```python
from build123d import *
from OCP.BRepFilletAPI import BRepFilletAPI_MakeChamfer

# Parameters (mm, degrees)
SKETCH1_R           = 3.96875
BOSS_EXTRUDE1_DEPTH = 12.7
SKETCH2_R           = 3.96875
CUT_EXTRUDE1_DEPTH  = 4.7625
SKETCH3_R           = 2.5796875
CUT_EXTRUDE2_DEPTH  = 34.474321177
CHAMFER1_SIZE       = 8.89
CHAMFER1_SIZE2      = 3.235695383


with BuildPart() as part:
    # Sketch1 → Boss-Extrude1 (new body)
    with BuildSketch(Plane(origin=(0, 0, 0), x_dir=(1, 0, 0), z_dir=(0, 1, 0))):
        Polygon((0, 0), (27.305, 0), (27.305, 19.3802), (0, 19.3802), (0, 14.6177), (14.605, 14.6177), (14.605, 4.7625), (0, 4.7625), align=None)
        with Locations(Location((20.955, 9.6901, 0), (0, 0, 270))):
            Circle(SKETCH1_R, mode=Mode.SUBTRACT)
    extrude(amount=BOSS_EXTRUDE1_DEPTH)

    # Sketch2 → Cut-Extrude1 (cut)
    with BuildSketch(Plane.XY):
        with Locations((6.985, 6.35)):
            Circle(SKETCH2_R)
    extrude(amount=-CUT_EXTRUDE1_DEPTH, mode=Mode.SUBTRACT)

    # Sketch3 → Cut-Extrude2 (cut, through all)
    with BuildSketch(Plane.XY.offset(-14.6177)):
        with Locations((6.985, 6.35)):
            Circle(SKETCH3_R)
    extrude(amount=-CUT_EXTRUDE2_DEPTH, mode=Mode.SUBTRACT)

    # Chamfer1: one chamfer whose edges measure the first distance from different faces: ONE call of the kernel's chamfer builder (chamfer() names one face for all edges)
    chamfer1_edges_1 = [part.edges().sort_by_distance(p)[0] for p in [
        (27.305, 6.35, -19.3802),
    ]]
    chamfer1_side_1 = [part.faces().sort_by_distance(p)[0] for p in [
        (14.080266617, 6.35, -19.3802),
    ]]
    chamfer1_edges_2 = [part.edges().sort_by_distance(p)[0] for p in [
        (27.305, 6.35, 0),
    ]]
    chamfer1_side_2 = [part.faces().sort_by_distance(p)[0] for p in [
        (14.762286847, 6.35, 0),
    ]]
    chamfer1 = BRepFilletAPI_MakeChamfer(part.part.solid().wrapped)
    for e in chamfer1_edges_1:
        chamfer1.Add(CHAMFER1_SIZE, CHAMFER1_SIZE2, e.wrapped, chamfer1_side_1[0].wrapped)  # the first distance lies on this face
    for e in chamfer1_edges_2:
        chamfer1.Add(CHAMFER1_SIZE, CHAMFER1_SIZE2, e.wrapped, chamfer1_side_2[0].wrapped)  # the first distance lies on this face
    add(Compound.cast(chamfer1.Shape()), mode=Mode.REPLACE)


solid = part.part
```
The listing builds one solid part. Answer for the finished solid, in the listing's coordinates (mm). A direction names the side the tool comes from. Give positions to 0.01 mm unless a question says otherwise; leave off trailing zeros. Order: outer loops, then holes, each group sorted by start corner. A loop starts at its lowest first (then second) coordinate and runs counter-clockwise, first axis right, second up. Notation, with made-up numbers: M -29,44 L -21,44 A22 ccw -21,65 Z; hole C -24.75,23.5 d5. An arc over 180 degrees is marked long. Put each result on its own line as item: value. Start each with the question number.
Item 1: The part is cut by section D-D, the plane x = 4. Determine the outline of the cut face in (y, z).
Item 2: For a pull along Y with two mould halves and no side action, classify faces 3 (the face through (10.77, 7.54, -2.35)), 4 (the face through (16, 0, -10)), 5 (the face through (9.3, 4.8, -19.38)) as +Y half, -Y half, draft (parallel to the pull), parting line (faces both ways), or undercut.
Item 3: The part is cut by section A-A, the plane y = 8.25. Determine the outline of the cut face in (x, z) (1 decimal).
Item 4: Which of the six approach directions +Z, -Z, +X, -X, +Y, -Y give full straight-line access (tool end or side, diameter ignored) to faces 1 (the face through (22.92, 6.26, -1.64)), 2 (the face through (7.2, 9.1, -14.618))?
Item 5: The part is cut by section B-B, the plane z = -8.75. Determine the outline of the cut face in (x, y) (3 decimals).
Item 6: Flat-ended cylindrical pins translate along their axes: P1, Ø3, axis at y = 7.5, z = -4, coming from the -X side; P2, Ø7, axis at x = 20.96, z = -9.69, coming from the +Y side; P3, Ø3, axis at y = 4, z = -12, coming from the -X side (3 decimals). Find the tip coordinate at first contact, or state that the pin passes through.
Item 7: Find the intervals of material crossed by line 1 along Z through (x, y) = (3.5, 2.5); line 2 along X through (y, z) = (3.75, -7.25) (3 decimals); line 3 along Z through (x, y) = (18, 8.25), in increasing order.
Answer key:
1. outline: M 0,-19.38 L 12.7,-19.38 L 12.7,-14.62 L 0,-14.62 Z; M 0,-4.76 L 3.73,-4.76 L 3.73,0 L 0,0 Z; M 8.97,-4.76 L 12.7,-4.76 L 12.7,0 L 8.97,0 Z
2. face 3: undercut
2. face 4: -Y half
2. face 5: draft
3. outline: M 0,-19.4 L 5.2,-19.4 L 5.2,-14.6 L 0,-14.6 Z; M 0,-4.8 L 3.5,-4.8 L 3.5,0 L 0,0 Z; M 8.7,-19.4 L 18.4,-19.4 L 27.3,-16.1 L 27.3,-3.2 L 18.4,0 L 10.5,0 L 10.5,-4.8 L 14.6,-4.8 L 14.6,-14.6 L 8.7,-14.6 Z; hole C 21,-9.7 d7.9
4. face 1: +Z, +X, +Y, -Y
4. face 2: -X, +Y, -Y
5. outline: M 14.605,0 L 17.099,0 L 17.099,12.7 L 14.605,12.7 Z; M 24.811,0 L 27.305,0 L 27.305,12.7 L 24.811,12.7 Z
6. P1: stops at x = 0
6. P2: passes through
6. P3: stops at x = 14.605
7. line 1: z = -19.38 to -14.62, -4.76 to 0
7. line 2: x = 14.605 to 17.825, 24.085 to 27.305
7. line 3: z = -19.38 to -12.34, -7.04 to 0
